Could you check a few things on this model? Use its own coordinates, in mm. A direction names the side the tool comes from. Coordinates: 2 decimals unless noted, no trailing zeros. Loops run counter-clockwise (first coordinate to the right, second up) from the corner with the lowest first, then second, coordinate; pieces in that order, holes last.
from build123d import *

# Parameters (mm, degrees)
SKIZZE1_W                       = 100
SKIZZE1_H                       = 60
AUFSATZ_LINEAR_AUSTRAGEN1_DEPTH = 460
SKIZZE2_W                       = 100
SKIZZE2_H                       = 100
SCHNITT_LINEAR_AUSTRAGEN1_DEPTH = 30


with BuildPart() as part:
    # Skizze1 → Aufsatz-Linear austragen1 (new, symmetric)
    with BuildSketch(Plane.XY):
        Rectangle(SKIZZE1_W, SKIZZE1_H)
    extrude(amount=AUFSATZ_LINEAR_AUSTRAGEN1_DEPTH, both=True)

    # Skizze2 → Schnitt-Linear austragen1 (cut)
    with BuildSketch(Plane(origin=(0, 30, 0), x_dir=(1, 0, 0), z_dir=(0, 1, 0))):
        Rectangle(SKIZZE2_W, SKIZZE2_H)
    extrude(amount=-SCHNITT_LINEAR_AUSTRAGEN1_DEPTH, mode=Mode.SUBTRACT)


solid = part.part
(1) Imagine slicing it at A-A, the plane x = 42.5. Write out the boundary of the cut face in (y, z), and give its area (3 significant figures).
Answers:
outline: (-30, -460) - (30, -460) - (30, -50) - (0, -50) - (0, 50) - (30, 50) - (30, 460) - (-30, 460) - close
area: 52,200 mm2
(2) We'd pull the mould along Z, two halves only. Please class faces 3 (the face through (-1, 0, -1)), 4 (the face through (-50, -0.4, 6.4)), 5 (the face through (-1, 0, 460)), 6 (the face through (-1, 0, -460)): +Z half, -Z half, draft (parallel to the pull), parting line (faces both ways), or undercut.
Answers:
face 3: undercut
face 4: draft
face 5: +Z half
face 6: -Z half
(3) Which directions (+Z, -Z, +X, -X, +Y, -Y) give clear straight access to the entire face, cutting with the end or side of a thin tool? Please do faces 1 (the face through (-1, 15, 50)), 2 (the face through (-1, 30, -252)).
Answers:
face 1: +X, -X, +Y
face 2: +Z, -Z, +X, -X, +Y
(4) I need wall thicknesses on probe 1 along Z at (x, y) = (-2, 10.5); probe 2 along Y at (x, z) = (13, 1). Which ranges of each line are inside material? Lowest first, please.
Answers:
probe 1: z = -460 to -50, 50 to 460
probe 2: y = -30 to 0
